The listing builds one solid part. Answer for the finished solid, in the listing's coordinates (mm). A direction names the side the tool comes from. Round coordinates to 2 decimals unless told otherwise and drop trailing zeros. Loops run counter-clockwise (first coordinate to the right, second up) from the corner with the lowest first, then second, coordinate; pieces in that order, holes last. Notation, with made-up numbers: (14.5, 9) -> (70.5, 9) arc R20 ccw to (70.5, 37) -> close; hole circle Ø7 at (-21, 10). An arc over 180 degrees is marked (long way). Use a Markdown table: item, result. Add a question column.
Q1. For a pull along X with two mould halves and no side action, classify faces 4 (the cylindrical face through (43.5, 10.07, 1.48)), 5 (the flat face through (25, 35.724, 2)), 6 (the flat face through (0, 25, 2)), 7 (the cylindrical face through (43.894, 31.738, 1.521)) as released by +X, released by -X, zero draft, split by the parting line, or undercut.
Q2. Section C-C on y = 3.5 is taken. Give the vertices of the cut face in (x, z), then the cut area to 3 significant figures.
Q3. Section A-A on y = 10 is taken. Give the vertices of the cut face in (x, z), then the cut area to 3 significant figures.
Q4. Which of the six approach directions +Z, -Z, +X, -X, +Y, -Y give full straight-line access (tool end or side, diameter ignored) to faces 1 (the cylindrical face through (-5.16, -8.76, 1.48)), 2 (the flat face through (41, 7, 2)), 3 (the flat face through (50, 25, 2))?
Q5. Given pin 1 Ø1.5 at (x, z) = (30.5, 1.5) entering from -Y; pin 2 Ø2.5 at (x, y) = (45, 30.72) entering from +Z, each flat-ended and moving along its own axis, determine where each tip first touches the part or whether it passes through.
Q6. Section D-D on x = 45 is taken. Give the vertices of the cut face in (y, z), then the cut area to 3 significant figures.
Q7. Section B-B on x = -5 is taken. Give the vertices of the cut face in (y, z).
Q8. Consider line 1 (X direction, y = 24, z = 2.8); line 2 (X direction, y = 31, z = 1.55); line 3 (X direction, y = 9.5, z = 2.05). Determine where each line is inside the solid, lowest interval first.
from build123d import *

# Parameters (mm, degrees)
SKETCH1_R           = 1.25
SKETCH1_R_2         = 1.5
BOSS_EXTRUDE1_DEPTH = 3
SKETCH2_R           = 1.5
BOSS_EXTRUDE2_DEPTH = 3
SKETCH3_W           = 32
SKETCH3_H           = 21.44761059
CUT_EXTRUDE1_DEPTH  = 4


with BuildPart() as part:
    # Sketch1 → Boss-Extrude1 (new body)
    with BuildSketch(Plane.XY):
        with BuildLine():
            Line((-9, 10.723805295), (-9, -10.723805295))
            ThreePointArc((-9, -10.723805295), (0, -14), (9, -10.723805295))
            Line((9, -10.723805295), (41, -10.723805295))
            ThreePointArc((41, -10.723805295), (50, -14), (59, -10.723805295))
            Line((59, -10.723805295), (59, 10.723805295))
            ThreePointArc((59, 10.723805295), (50, 14), (41, 10.723805295))
            Line((41, 10.723805295), (9, 10.723805295))
            ThreePointArc((9, 10.723805295), (0, 14), (-9, 10.723805295))
        make_face()
        Circle(SKETCH1_R, mode=Mode.SUBTRACT)
        with Locations((-5, 10)):
            Circle(SKETCH1_R, mode=Mode.SUBTRACT)
        with Locations((5, 10)):
            Circle(SKETCH1_R, mode=Mode.SUBTRACT)
        with Locations((-5, -10)):
            Circle(SKETCH1_R, mode=Mode.SUBTRACT)
        with Locations((5, -10)):
            Circle(SKETCH1_R, mode=Mode.SUBTRACT)
        with Locations((50, 0)):
            Circle(SKETCH1_R, mode=Mode.SUBTRACT)
        with Locations((45, 10)):
            Circle(SKETCH1_R_2, mode=Mode.SUBTRACT)
        with Locations((55, 10)):
            Circle(SKETCH1_R_2, mode=Mode.SUBTRACT)
        with Locations((45, -10)):
            Circle(SKETCH1_R_2, mode=Mode.SUBTRACT)
        with Locations((55, -10)):
            Circle(SKETCH1_R_2, mode=Mode.SUBTRACT)
        with Locations((25, 0)):
            Circle(SKETCH1_R, mode=Mode.SUBTRACT)
        with Locations((25, 5)):
            Circle(SKETCH1_R, mode=Mode.SUBTRACT)
        with Locations((25, -5)):
            Circle(SKETCH1_R, mode=Mode.SUBTRACT)
        with Locations((35, 0)):
            Circle(SKETCH1_R, mode=Mode.SUBTRACT)
        with Locations((15, 0)):
            Circle(SKETCH1_R, mode=Mode.SUBTRACT)
        with Locations((35, 5)):
            Circle(SKETCH1_R, mode=Mode.SUBTRACT)
        with Locations((35, -5)):
            Circle(SKETCH1_R, mode=Mode.SUBTRACT)
        with Locations((15, -5)):
            Circle(SKETCH1_R, mode=Mode.SUBTRACT)
        with Locations((15, 5)):
            Circle(SKETCH1_R, mode=Mode.SUBTRACT)
    extrude(amount=BOSS_EXTRUDE1_DEPTH)

    # Sketch2 → Boss-Extrude2 (add)
    with BuildSketch(Plane.XY.offset(3)):
        with BuildLine():
            Line((0, 14), (0, 35.723805295))
            Line((0, 35.723805295), (50, 35.723805295))
            Line((50, 35.723805295), (50, 14))
            ThreePointArc((50, 14), (45.21112091, 13.155479355), (41, 10.723805295))
            Line((41, 10.723805295), (41, 25.723805295))
            Line((41, 25.723805295), (9, 25.723805295))
            Line((9, 25.723805295), (9, 10.723805295))
            ThreePointArc((9, 10.723805295), (4.78887909, 13.155479355), (0, 14))
        make_face()
        with Locations((5, 30.723805295)):
            Circle(SKETCH2_R, mode=Mode.SUBTRACT)
        with Locations((45, 30.723805295)):
            Circle(SKETCH2_R, mode=Mode.SUBTRACT)
        with Locations((45, 20.723805295)):
            Circle(SKETCH2_R, mode=Mode.SUBTRACT)
        with Locations((5, 20.723805295)):
            Circle(SKETCH2_R, mode=Mode.SUBTRACT)
    extrude(amount=-BOSS_EXTRUDE2_DEPTH)

    # Sketch3 → Cut-Extrude1 (cut, through all)
    with BuildSketch(Plane.XY.offset(3)):
        with Locations((25, 0)):
            Rectangle(SKETCH3_W, SKETCH3_H)
    extrude(amount=-CUT_EXTRUDE1_DEPTH, mode=Mode.SUBTRACT)


solid = part.part
Checked values:
| question | item | result |
|---|---|---|
| 1 | face 4 | undercut |
| 1 | face 5 | zero draft |
| 1 | face 6 | released by -X |
| 1 | face 7 | undercut |
| 2 | outline | (-9, 0) -> (9, 0) -> (9, 3) -> (-9, 3) -> close; (41, 0) -> (59, 0) -> (59, 3) -> (41, 3) -> close |
| 2 | area | 108 mm2 |
| 3 | outline | (-9, 0) -> (-6.25, 0) -> (-6.25, 3) -> (-9, 3) -> close; (-3.75, 0) -> (3.75, 0) -> (3.75, 3) -> (-3.75, 3) -> close; (6.25, 0) -> (9, 0) -> (9, 3) -> (6.25, 3) -> close; (41, 0) -> (43.5, 0) -> (43.5, 3) -> (41, 3) -> close; (46.5, 0) -> (53.5, 0) -> (53.5, 3) -> (46.5, 3) -> close; (56.5, 0) -> (59, 0) -> (59, 3) -> (56.5, 3) -> close |
| 3 | area | 75.0 mm2 |
| 4 | face 1 | +Z, -Z |
| 4 | face 2 | +Z, -Z, -Y |
| 4 | face 3 | +Z, -Z, +X, +Y |
| 5 | pin 1 | stops at y = 25.72 |
| 5 | pin 2 | passes through |
| 6 | outline | (-13.08, 0) -> (-11.5, 0) -> (-11.5, 3) -> (-13.08, 3) -> close; (-8.5, 0) -> (8.5, 0) -> (8.5, 3) -> (-8.5, 3) -> close; (11.5, 0) -> (19.22, 0) -> (19.22, 3) -> (11.5, 3) -> close; (22.22, 0) -> (29.22, 0) -> (29.22, 3) -> (22.22, 3) -> close; (32.22, 0) -> (35.72, 0) -> (35.72, 3) -> (32.22, 3) -> close |
| 6 | area | 110 mm2 |
| 7 | outline | (-13.08, 0) -> (-11.25, 0) -> (-11.25, 3) -> (-13.08, 3) -> close; (-8.75, 0) -> (8.75, 0) -> (8.75, 3) -> (-8.75, 3) -> close; (11.25, 0) -> (13.08, 0) -> (13.08, 3) -> (11.25, 3) -> close |
| 8 | line 1 | x = 0 to 9, 41 to 50 |
| 8 | line 2 | x = 0 to 3.53, 6.47 to 43.53, 46.47 to 50 |
| 8 | line 3 | x = -9 to -6.15, -3.85 to 3.85, 6.15 to 9, 41 to 43.59, 46.41 to 53.59, 56.41 to 59 |
